Autodesk Inventor part; units mm, degrees
ref_plane "YZ Plane" through (0, 0, 0) normal (1, 0, 0) x (0, 1, 0)
ref_plane "XZ Plane" through (0, 0, 0) normal (0, 1, 0) x (-1, 0, 0)
ref_plane "XY Plane" through (0, 0, 0) normal (0, 0, 1) x (1, 0, 0)
sketch "Sketch1" plane through (0, 0, 0) normal (0, 0, 1) x (1, 0, 0)
  line L0 (-20, -40) -> (20, -40)
  line L1 (20, -40) -> (20, 40)
  line L2 (20, 40) -> (-20, 40)
  line L3 (-20, 40) -> (-20, -40)
  line L4 (-20, -40) -> (20, 40) construction
  line L5 (20, -40) -> (-20, 40) construction
  line L6 (-5, 40) -> (5, 40)
  line L7 (5, 40) -> (5, 25)
  line L8 (5, 25) -> (-5, 25)
  line L9 (-5, 25) -> (-5, 40)
  line L10 (0, 40) -> (0, 0)
  dimension "d0" = 40
  dimension "d1" = 80
  dimension "d2" = 15
  dimension "d3" = 10
extrude "Plate1" add sketch "Sketch1" along normal blind 3 contours L3 L2 L9 L8 L7 L1 L0
equation "\"d4\" = Thickness"
equation "\"BendRadius\" = Thickness"
equation "\"BendReliefWidth\" = Thickness"
equation "\"BendReliefDepth\" = 0.5 * Thickness"
equation "\"CornerReliefSize\" = 4 * Thickness"
equation "\"MinimumRemnant\" = 2 * Thickness"
equation "\"TransitionRadius\" = BendRadius"
equation "\"JacobiRadiusSize\" = BendRadius"
equation "\"GapSize\" = Thickness"
properties part number "ramp extension"
Source: CAD feature listing. Evaluate the final solid. Frame: model axes, mm. A direction names the side the tool comes from. Round coordinates to 2 decimals unless told otherwise and drop trailing zeros. Order: outer loops, then holes, each group sorted by start corner. A loop starts at its lowest first (then second) coordinate and runs counter-clockwise, first axis right, second up. Notation, with made-up numbers: (9.25, 72.5) -> (55.25, 72.5) arc R29 cw to (55.25, 98.5) -> close; hole circle Ø10 at (82.25, 4.25). An arc over 180 degrees is marked (long way). Answer as CSV lines item,"result".
Item 1: Line query: L1, parallel to X at y = 30, z = 1.9; L2, parallel to Y at x = -2, z = 1.35. Output: solid intervals per line, ascending.
A:
L1,"-20 to -5, 5 to 20"
L2,"-40 to 25"
Item 2: Section B-B, the plane z = 1.95. Return loops of the section in (x, y), plus the area to 3 significant figures.
A:
outline,"(-20, -40) -> (20, -40) -> (20, 40) -> (5, 40) -> (5, 25) -> (-5, 25) -> (-5, 40) -> (-20, 40) -> close"
area,"3,050 mm²"
Item 3: Pull-direction query (X, two-part tool) for faces 3 (the face through (-20, 1, 1)), 4 (the face through (13, 40, 1)), 5 (the face through (0, 25, 1)); classes: pulls with the +X half, pulls with the -X half, needs draft (parallel to the pull), parting line crosses it, or undercut.
A:
face 3,"pulls with the -X half"
face 4,"needs draft"
face 5,"undercut"
Item 4: Reachability of faces 1 (the face through (-12, 40, 1)), 2 (the face through (5, 33, 1)) from +Z, -Z, +X, -X, +Y, -Y: full face, straight path, thin tool, end or side. Return the list, or none.
A:
face 1,"+Z, -Z, +X, -X, +Y"
face 2,"+Z, -Z, +Y"
Item 5: Section C-C, the plane x = 3. Return loops of the section in (y, z).
A:
outline,"(-40, 0) -> (25, 0) -> (25, 3) -> (-40, 3) -> close"
Item 6: Section A-A, the plane y = 26. Return loops of the section in (x, z).
A:
outline,"(-20, 0) -> (-5, 0) -> (-5, 3) -> (-20, 3) -> close; (5, 0) -> (20, 0) -> (20, 3) -> (5, 3) -> close"
Item 7: Pin query (flat end, axial travel): pin 1 Ø0.9 at (x, z) = (2, 1.5) entering from +Y. Return the tip coordinate at first contact, or that it passes through.
A:
pin 1,"y = 25"
